from build123d import *

# Parameters (mm, degrees)
BASE_FLANGE1_DEPTH = 16
SKETCH8_R          = 1.25
CUT_EXTRUDE1_DEPTH = 2


# Sheet-metal steps are written as plain solids
with BuildPart() as part:
    # Sketch1 → Base-Flange1 (new body)
    with BuildSketch(Plane.XY):
        with BuildLine():
            Line((-13.822681927, 15.418198529), (-13.822681927, 9.918198529))
            ThreePointArc((-13.822681927, 9.918198529), (-12.358215833, 6.382664623), (-8.822681927, 4.918198529))
            Line((-8.822681927, 4.918198529), (11.677318073, 4.918198529))
            ThreePointArc((11.677318073, 4.918198529), (15.212851979, 6.382664623), (16.677318073, 9.918198529))
            Line((16.677318073, 9.918198529), (16.677318073, 15.418198529))
            Line((16.677318073, 15.418198529), (14.677318073, 15.418198529))
            Line((14.677318073, 15.418198529), (14.677318073, 9.918198529))
            ThreePointArc((14.677318073, 9.918198529), (13.798638417, 7.796878186), (11.677318073, 6.918198529))
            Line((11.677318073, 6.918198529), (-8.822681927, 6.918198529))
            ThreePointArc((-8.822681927, 6.918198529), (-10.94400227, 7.796878186), (-11.822681927, 9.918198529))
            Line((-11.822681927, 9.918198529), (-11.822681927, 15.418198529))
            Line((-11.822681927, 15.418198529), (-13.822681927, 15.418198529))
        make_face()
    extrude(amount=BASE_FLANGE1_DEPTH)

    # Sketch8 → Cut-Extrude1 (cut)
    with BuildSketch(Plane(origin=(0, 6.918198529, 0), x_dir=(1, 0, 0), z_dir=(0, 1, 0))):
        with Locations(Location((3.992812071, -8.013954427, 0), (0, 0, 270))):
            Circle(SKETCH8_R)
        with Locations(Location((-1.122681927, -8, 0), (0, 0, 270))):
            Circle(SKETCH8_R)
    extrude(amount=-CUT_EXTRUDE1_DEPTH, mode=Mode.SUBTRACT)


solid = part.part
Build history of the part. All positions in model axes, mm. A direction names the side the tool comes from. Round coordinates to 2 decimals unless told otherwise and drop trailing zeros. Write each loop counter-clockwise with the first axis right and the second up, starting at its lowest first coordinate (ties: lowest second). Pieces come first, ordered by that corner, then holes. Notation, with made-up numbers: (2.5, 2.5) -> (61.5, 2.5) arc R38 ccw to (61.5, 40.5) -> close; hole circle Ø11 at (49, -0.75). An arc over 180 degrees is marked (long way). Use one line per item in the form item = value.
Q1. Band-saw the part on B-B, the plane z = 8.25. Write the cut outline in (x, y), then the cut area to 3 significant figures.
Conclusion:
outline = (-13.82, 9.92) arc R5 ccw to (-8.82, 4.92) -> (-2.35, 4.92) -> (-2.35, 6.92) -> (-8.82, 6.92) arc R3 cw to (-11.82, 9.92) -> (-11.82, 15.42) -> (-13.82, 15.42) -> close; (0.1, 4.92) -> (2.77, 4.92) -> (2.77, 6.92) -> (0.1, 6.92) -> close; (5.22, 4.92) -> (11.68, 4.92) arc R5 ccw to (16.68, 9.92) -> (16.68, 15.42) -> (14.68, 15.42) -> (14.68, 9.92) arc R3 cw to (11.68, 6.92) -> (5.22, 6.92) -> close
area = 78.3 mm²
Q2. Two-plate mould, pull along Z, no slides. Class faces 3 (the flat face through (1.2, 6.7, 0)), 4 (the cylindrical face through (3.514, 5.932, 9.169)), 5 (the cylindrical face through (-12.397, 6.422, 7.888)): released by +Z, released by -Z, zero draft, split by the parting line, or undercut.
Conclusion:
face_3 = released by -Z
face_4 = undercut
face_5 = zero draft
Q3. Drill centre lines: L1, parallel to X at y = 9.75, z = 13.5; L2, parallel to X at y = 5.95, z = 8; L3, parallel to Y at x = 8, z = 12.25. Where is each one in solid material? Low to high.
Conclusion:
L1 = -13.82 to -11.82, 14.67 to 16.67
L2 = -11.86 to -2.37, 0.13 to 2.74, 5.24 to 14.72
L3 = 4.92 to 6.92
Q4. Band-saw the part on A-A, the plane x = -1.5. Write the cut outline in (y, z), then the cut area to 3 significant figures.
Conclusion:
outline = (4.92, 0) -> (6.92, 0) -> (6.92, 6.81) -> (4.92, 6.81) -> close; (4.92, 9.19) -> (6.92, 9.19) -> (6.92, 16) -> (4.92, 16) -> close
area = 27.2 mm²
Q5. Band-saw the part on D-D, the plane x = -6.5. Write the cut outline in (y, z).
Conclusion:
outline = (4.92, 0) -> (6.92, 0) -> (6.92, 16) -> (4.92, 16) -> close
Q6. Tool access for faces 1 (the flat face through (14.677, 13, 8)), 2 (the flat face through (16.677, 13, 8)): list every direction of +Z, -Z, +X, -X, +Y, -Y with a clear straight run to the whole face (end or side of a thin tool).
Conclusion:
face_1 = +Z, -Z, +Y
face_2 = +Z, -Z, +X, +Y, -Y
Q7. Band-saw the part on C-C, the plane z = 4. Write the cut outline in (x, y), then the cut area to 3 significant figures.
Conclusion:
outline = (-13.82, 9.92) arc R5 ccw to (-8.82, 4.92) -> (11.68, 4.92) arc R5 ccw to (16.68, 9.92) -> (16.68, 15.42) -> (14.68, 15.42) -> (14.68, 9.92) arc R3 cw to (11.68, 6.92) -> (-8.82, 6.92) arc R3 cw to (-11.82, 9.92) -> (-11.82, 15.42) -> (-13.82, 15.42) -> close
area = 88.1 mm²
Q8. Drop flat-ended pins along their axis: P1, Ø1, axis at x = -10.5, z = 5.5, coming from the +Y side; P2, Ø1.5, axis at x = -1.12, z = 8, coming from the -Y side; P3, Ø6, axis at x = 10.5, z = 5.5, coming from the +Y side. Give the stop position or say it passes through.
Conclusion:
P1 = 7.85
P2 = through
P3 = 7.54
